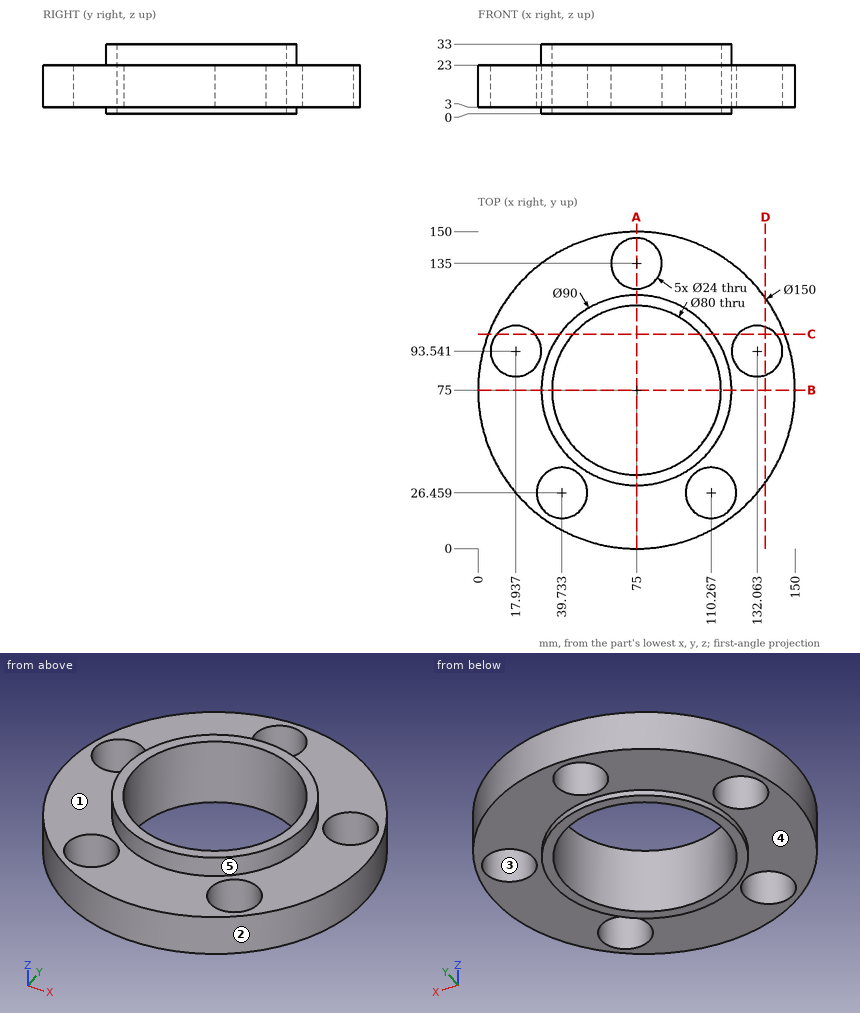
Study the drawing (mm; zero at the part's minimum x, y, z) and answer. A direction names the side the tool comes from. Give positions to 0.01 mm unless a question says otherwise; leave off trailing zeros. Write each loop counter-clockwise with the first axis right and the second up, starting at its lowest first coordinate (ties: lowest second). Pieces come first, ordered by that corner, then holes. Notation, with made-up numbers: (33.25, 9.25) -> (65.25, 9.25) arc R14 cw to (65.25, 19.25) -> close; hole circle Ø3 at (71.25, -20). An arc over 180 degrees is marked (long way). Answer in a Markdown table with one row per item.
1) Section C-C on y = 101.5 is taken. Give the vertices of the cut face in (x, z), plus the area to 3 significant figures.
Results list:
| item | result |
|---|---|
| outline | (4.84, 3) -> (8.96, 3) -> (8.96, 23) -> (4.84, 23) -> close; (26.92, 3) -> (38.63, 3) -> (38.63, 0) -> (45.04, 0) -> (45.04, 33) -> (38.63, 33) -> (38.63, 23) -> (26.92, 23) -> close; (104.96, 0) -> (111.37, 0) -> (111.37, 3) -> (123.08, 3) -> (123.08, 23) -> (111.37, 23) -> (111.37, 33) -> (104.96, 33) -> close; (141.04, 3) -> (145.16, 3) -> (145.16, 23) -> (141.04, 23) -> close |
| area | 1,060 mm^2 |
2) Section D-D on x = 136 is taken. Give the vertices of the cut face in (y, z) (1 decimal).
Results list:
| item | result |
|---|---|
| outline | (31.4, 3) -> (82.2, 3) -> (82.2, 23) -> (31.4, 23) -> close; (104.9, 3) -> (118.6, 3) -> (118.6, 23) -> (104.9, 23) -> close |
3) Determine the mould class of the marked faces 3, 4 and 5 for opening direction Y: released by +Y, released by -Y, zero draft, split by the parting line, or undercut.
Results list:
| item | result |
|---|---|
| face 3 | undercut |
| face 4 | zero draft |
| face 5 | split by the parting line |
4) Straight lines are drawn through the part: line 1 (Y direction, x = 75, z = 16.25); line 2 (X direction, y = 32, z = 4.5); line 3 (X direction, y = 75.5, z = 5.5). For each, find the intervals that lie inside material, in ascending order. Write a range as [from, to].
Results list:
| item | result |
|---|---|
| line 1 | [0, 35], [115, 123], [147, 150] |
| line 2 | [13.55, 29.09], [50.38, 99.62], [120.91, 136.45] |
| line 3 | [0, 35], [115, 150] |
5) A tool of negligible diameter and unlimited length cuts with its end or side. For the marked faces 1 and 2, from which of +Z, -Z, +X, -X, +Y, -Y can it reach the whole face along a straight path? Write none if from no direction.
Results list:
| item | result |
|---|---|
| face 1 | +Z |
| face 2 | +Z, -Z |
6) Each of these flat-tipped pins is pushed along its axis until it touches: pin 1 Ø4 at (x, z) = (105, 12.5) entering from -Y; pin 2 Ø4 at (x, z) = (81, 28) entering from -Y; pin 3 Ø2 at (x, z) = (86, 6) entering from -Y. Where does it stop, or does it pass through?
Results list:
| item | result |
|---|---|
| pin 1 | y = 5.42 |
| pin 2 | y = 30.18 |
| pin 3 | y = 0.67 |
7) Section B-B on y = 75 is taken. Give the vertices of the cut face in (x, z), plus the area to 3 significant figures.
Results list:
| item | result |
|---|---|
| outline | (0, 3) -> (30, 3) -> (30, 0) -> (35, 0) -> (35, 33) -> (30, 33) -> (30, 23) -> (0, 23) -> close; (115, 0) -> (120, 0) -> (120, 3) -> (150, 3) -> (150, 23) -> (120, 23) -> (120, 33) -> (115, 33) -> close |
| area | 1,530 mm^2 |
8) Section A-A on x = 75 is taken. Give the vertices of the cut face in (y, z), plus the area to 3 significant figures.
Results list:
| item | result |
|---|---|
| outline | (0, 3) -> (30, 3) -> (30, 0) -> (35, 0) -> (35, 33) -> (30, 33) -> (30, 23) -> (0, 23) -> close; (115, 0) -> (120, 0) -> (120, 3) -> (123, 3) -> (123, 23) -> (120, 23) -> (120, 33) -> (115, 33) -> close; (147, 3) -> (150, 3) -> (150, 23) -> (147, 23) -> close |
| area | 1,050 mm^2 |
